Input: part model. Units: mm. Frame: model coordinates. A direction names the side the tool comes from. Give positions to 0.01 mm unless a question says otherwise; leave off trailing zeros. Write each loop counter-clockwise with the first axis right and the second up, starting at its lowest first coordinate (ties: lowest second). Pieces come first, ordered by that corner, then holes.
```python
from build123d import *

# Parameters (mm, degrees)
BOSS_EXTRU_1_DEPTH      = 250
ENL_V_MAT_EXTRU_1_DEPTH = 266.518360947


with BuildPart() as part:
    # Esquisse2 → Boss.-Extru.1 (new body)
    with BuildSketch(Plane.XY):
        with BuildLine():
            Line((2, 0), (78, 0))
            ThreePointArc((78, 0), (79.414213562, 0.585786438), (80, 2))
            Line((80, 2), (80, 38))
            ThreePointArc((80, 38), (79.414213562, 39.414213562), (78, 40))
            Line((78, 40), (2, 40))
            ThreePointArc((2, 40), (0.585786438, 39.414213562), (0, 38))
            Line((0, 38), (0, 2))
            ThreePointArc((0, 2), (0.585786438, 0.585786438), (2, 0))
        make_face()
        with BuildLine():
            Line((6, 4), (74, 4))
            ThreePointArc((74, 4), (75.414213562, 4.585786438), (76, 6))
            Line((76, 6), (76, 34))
            ThreePointArc((76, 34), (75.414213562, 35.414213562), (74, 36))
            Line((74, 36), (6, 36))
            ThreePointArc((6, 36), (4.585786438, 35.414213562), (4, 34))
            Line((4, 34), (4, 6))
            ThreePointArc((4, 6), (4.585786438, 4.585786438), (6, 4))
        make_face(mode=Mode.SUBTRACT)
    extrude(amount=BOSS_EXTRU_1_DEPTH)

    # Esquisse3 → Enlèv. mat.-Extru.1 (cut, through all)
    with BuildSketch(Plane(origin=(80, 0, 0), x_dir=(0, 0, -1), z_dir=(1, 0, 0))):
        Polygon((0, 25), (-25, 0), (0, 0), align=None)
        Polygon((-250, 25), (-225, 0), (-250, 0), align=None)
    extrude(amount=-ENL_V_MAT_EXTRU_1_DEPTH, mode=Mode.SUBTRACT)


solid = part.part
```
Q1. Access query for faces 1 (the flat face through (41, 40, 123)), 2 (the flat face through (40, 4, 124)). Directions: +Z, -Z, +X, -X, +Y, -Y. A direction counts if a zero-diameter tool reaches every point of the face in a straight line with its end or side. Return the directions, or none.
Q2. Section B-B, the plane z = 138. Return the cut outline in (x, y), then the cut area to 3 significant figures.
Q3. Section A-A, the plane y = 22. Return the cut outline in (x, z).
Q4. Mould query, pull axis X, two halves, no side actions, for faces 3 (the flat face through (40, 37, 0)), 4 (the flat face through (0, 20, 123)), 5 (the flat face through (76, 20, 123)). Classes: +X half, -X half, draft (parallel to the pull), parting line (faces both ways), or undercut.
Q5. Material intervals for line 1 along X through (y, z) = (24, 235.5); line 2 along Y through (x, z) = (21, 185); line 3 along Y through (x, z) = (14, 22), sorted ascending.
Q6. Section C-C, the plane x = 41. Return the cut outline in (y, z).
Solutions:
1. face 1: +Z, -Z, +X, -X, +Y
1. face 2: +Z, -Z
2. outline: (0, 2) arc R2 ccw to (2, 0) - (78, 0) arc R2 ccw to (80, 2) - (80, 38) arc R2 ccw to (78, 40) - (2, 40) arc R2 ccw to (0, 38) - close; hole (4, 6) arc R2 ccw to (6, 4) - (74, 4) arc R2 ccw to (76, 6) - (76, 34) arc R2 ccw to (74, 36) - (6, 36) arc R2 ccw to (4, 34) - close
2. area: 896 mm2
3. outline: (0, 3) - (4, 3) - (4, 247) - (0, 247) - close; (76, 3) - (80, 3) - (80, 247) - (76, 247) - close
4. face 3: draft
4. face 4: -X half
4. face 5: undercut
5. line 1: x = 0 to 4, 76 to 80
5. line 2: y = 0 to 4, 36 to 40
5. line 3: y = 3 to 4, 36 to 40
6. outline: (0, 25) - (4, 21) - (4, 229) - (0, 225) - close; (36, 0) - (40, 0) - (40, 250) - (36, 250) - close
